Work out the finished part from the listing and answer in its coordinate system (mm). A direction names the side the tool comes from. Round coordinates to 2 decimals unless told otherwise and drop trailing zeros. Order: outer loops, then holes, each group sorted by start corner. A loop starts at its lowest first (then second) coordinate and runs counter-clockwise, first axis right, second up. Notation, with made-up numbers: (-14.5, -10) - (35.5, -10) arc R15 ccw to (35.5, 8) - close; hole circle Ø1 at (43, -36). An arc over 180 degrees is marked (long way). Answer in a Markdown table with one row per item.
from build123d import *

# Parameters (mm, degrees)
SKETCH3_OUTSIDE_W   = 19.328
SKETCH3_OUTSIDE_H   = 19.328
SKETCH3_OUTSIDE_W_2 = 6
SKETCH3_OUTSIDE_H_2 = 2.5
CUT_EXTRUDE2_DEPTH  = 60
SKETCH5_OUTSIDE_W   = 19.328
SKETCH5_OUTSIDE_H   = 19.328
SKETCH5_OUTSIDE_W_2 = 2.5
SKETCH5_OUTSIDE_H_2 = 6
CUT_EXTRUDE3_DEPTH  = 29


with BuildPart() as part:
    # Sketch2 → Revolve1 (revolve)
    with BuildSketch(Plane(origin=(0, 0, 0), x_dir=(1, 0, 0), z_dir=(0, 1, 0))):
        with BuildLine():
            Line((-27, 0), (-28, 0))
            ThreePointArc((-28, 0), (-26.070466269, -2.802517077), (-22.763932023, -2))
            Line((-22.763932023, -2), (0, -2))
            Line((0, -2), (0, 0))
            Line((0, 0), (-23, 0))
            ThreePointArc((-23, 0), (-25, -2), (-27, 0))
        make_face()
        with BuildLine():
            Line((0, 0), (0, -2))
            Line((0, -2), (22.763932023, -2))
            ThreePointArc((22.763932023, -2), (26.070466269, -2.802517077), (28, 0))
            Line((28, 0), (27, 0))
            ThreePointArc((27, 0), (25, -2), (23, 0))
            Line((23, 0), (0, 0))
        make_face()
    revolve(axis=Axis((0, 0, 0), (-1, 0, 0)))

    # Sketch3 outside → Cut-Extrude2 (cut)
    with BuildSketch(Plane(origin=(0, 0, 0), x_dir=(0, 0, -1), z_dir=(1, 0, 0))):
        Rectangle(SKETCH3_OUTSIDE_W, SKETCH3_OUTSIDE_H)
        Rectangle(SKETCH3_OUTSIDE_W_2, SKETCH3_OUTSIDE_H_2, mode=Mode.SUBTRACT)
    extrude(amount=-CUT_EXTRUDE2_DEPTH, mode=Mode.SUBTRACT)

    # Sketch5 outside → Cut-Extrude3 (cut, through all)
    with BuildSketch(Plane(origin=(0, 0, 0), x_dir=(0, 0, -1), z_dir=(1, 0, 0))):
        Rectangle(SKETCH5_OUTSIDE_W, SKETCH5_OUTSIDE_H)
        Rectangle(SKETCH5_OUTSIDE_W_2, SKETCH5_OUTSIDE_H_2, mode=Mode.SUBTRACT)
    extrude(amount=CUT_EXTRUDE3_DEPTH, mode=Mode.SUBTRACT)


solid = part.part
1) Find the intervals of material crossed by probe 1 along X at (y, z) = (-0.1, 0.15); probe 2 along X at (y, z) = (-0.7, 1); probe 3 along Z at (x, y) = (7, 0.55), in increasing order. Write a range as from..to.
Filled in:
| item | result |
|---|---|
| probe 1 | x = -27.99..-26.99, -23.01..23.01, 26.99..27.99 |
| probe 2 | x = -27.74..-26.58, -23.42..23.42, 26.58..27.74 |
| probe 3 | z = -1.25..1.25 |
2) Which of the six approach directions +Z, -Z, +X, -X, +Y, -Y give full straight-line access (tool end or side, diameter ignored) to faces 1 (the face through (-14, 1.25, 0)), 2 (the face through (14, 0, -1.25)), 3 (the face through (-11, 0, 2))?
Filled in:
| item | result |
|---|---|
| face 1 | +Z, -Z, -X, +Y |
| face 2 | -Z, +X, +Y, -Y |
| face 3 | +Z, +X |
3) Each of these flat-tipped pins is pushed along its axis until it touches: pin 1 (2 mm diameter, centred on x = -6, z = 2, fed in from +Y); pin 2 (3 mm diameter, centred on x = 14, z = 0.5, fed in from -Y); pin 3 (2 mm diameter, centred on y = -1, z = -1, fed in from +X). Where does it stop, or does it pass through?
Filled in:
| item | result |
|---|---|
| pin 1 | stops at y = 1.25 |
| pin 2 | stops at y = -2 |
| pin 3 | stops at x = 27.97 |
4) Find section B-B, the plane x = 10.5. Give the vertices of the cut face in (y, z).
Filled in:
| item | result |
|---|---|
| outline | (-1.56, -1.25) - (1.56, -1.25) arc R2 ccw to (1.56, 1.25) - (-1.56, 1.25) arc R2 ccw to start |
5) Find section A-A, the plane y = 0.65. Give the vertices of the cut face in (x, z), then the cut area to 3 significant figures.
Filled in:
| item | result |
|---|---|
| outline | (-22.76, -1.89) - (0, -1.89) - (0, -1.25) - (23.58, -1.25) arc R1.89 cw to (23.58, 1.25) - (0, 1.25) - (0, 1.89) - (-22.76, 1.89) arc R2.93 ccw (long way) to start; (26.42, -1.25) - (27.65, -1.25) arc R2.93 ccw to (27.65, 1.25) - (26.42, 1.25) arc R1.89 cw to start; hole circle Ø3.78 at (-25, 0) |
| area | 161 mm^2 |
